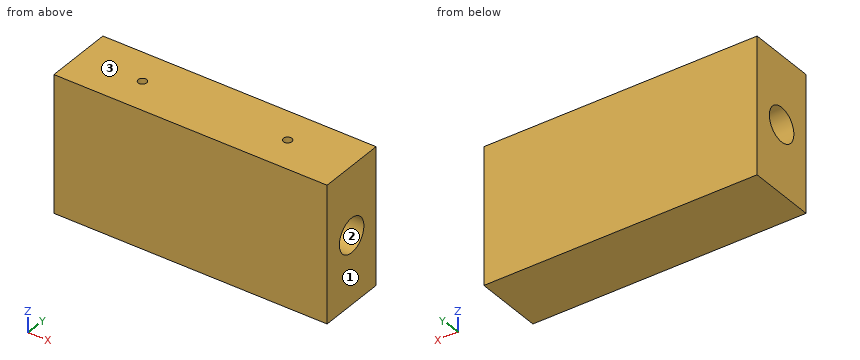
```python
from build123d import *

# Parameters (mm, degrees)
F0_W     = 101.6
F0_H     = 25.4
F1_DEPTH = 50.8
F3_D     = 3.175
F3_DEPTH = 12.7
F3_TIP   = 0.9538662327
F5_D     = 12.7


with BuildPart() as f1:
    # F0 (on Top) → F1 (new body)
    with BuildSketch(Plane.XY):
        Rectangle(F0_W, F0_H)
    extrude(amount=F1_DEPTH)

    # F3
    with Locations(Plane.XY.offset(50.8)):
        with Locations((-26.9875, 0), (26.9875, 0)):
            Hole(F3_D / 2, depth=F3_DEPTH)
            with Locations((0, 0, -(F3_DEPTH + F3_TIP / 2))):  # 118° drill point
                Cone(0, F3_D / 2, F3_TIP, mode=Mode.SUBTRACT)

    # F5 (through all)
    with Locations(Plane(origin=(-50.8, 0, 0), x_dir=(0, -1, 0), z_dir=(-1, 0, 0))):
        with Locations((0, 25.4)):
            Hole(F5_D / 2)


solid = f1.part
```
Work out the finished part from the listing and answer in its coordinate system (mm). Face numbers are marked on the shaded views. Coordinates: 2 decimals unless noted, no trailing zeros. Write each loop counter-clockwise with the first axis right and the second up, starting at its lowest first coordinate (ties: lowest second). Pieces come first, ordered by that corner, then holes. Notation, with made-up numbers: (64.25, 41) - (89.25, 41) arc R19 ccw to (89.25, 65) - close; hole circle Ø11 at (55.5, 2.5). An arc over 180 degrees is marked (long way). Answer as a JSON object with one key per item and string values.
Q1. Find section A-A (z = 25.4). Write down the section's boundary in (x, y).
Results list:
{"outline": "(-50.8, -12.7) - (50.8, -12.7) - (50.8, -6.35) - (-50.8, -6.35) - close; (-50.8, 6.35) - (50.8, 6.35) - (50.8, 12.7) - (-50.8, 12.7) - close"}
Q2. For a pull along Z with two mould halves and no side action, classify the marked faces 1, 2 and 3 as pulls with the +Z half, pulls with the -Z half, needs draft (parallel to the pull), parting line crosses it, or undercut.
Results list:
{"face 1": "needs draft", "face 2": "undercut", "face 3": "pulls with the +Z half"}
Q3. Find section B-B (x = 37). Write down the section's boundary in (y, z).
Results list:
{"outline": "(-12.7, 0) - (12.7, 0) - (12.7, 50.8) - (-12.7, 50.8) - close; hole circle Ø12.7 at (0, 25.4)"}
Q4. Given pin 1 Ø5 at (x, y) = (26.99, 0) entering from +Z; pin 2 Ø11.5 at (y, z) = (0, 25.4) entering from +X, each flat-ended and moving along its own axis, determine where each tip first touches the part or whether it passes through.
Results list:
{"pin 1": "stops at z = 50.8", "pin 2": "passes through"}
Q5. Consider L1, parallel to X at y = 0, z = 44.25 (3 decimals); L2, parallel to Z at x = 30, y = 0; L3, parallel to Y at x = 7, z = 25. Determine where each line is inside the solid, lowest interval first. Write a range as from..to.
Results list:
{"L1": "x = -50.8..-28.575, -25.4..25.4, 28.575..50.8", "L2": "z = 0..19.05, 31.75..50.8", "L3": "y = -12.7..-6.34, 6.34..12.7"}
